Could you check a few things on this model? Use its own coordinates, in mm. Face numbers are marked on the shaded views. A direction names the side the tool comes from. Give positions to 0.01 mm unless a question says otherwise; leave off trailing zeros. Write each loop counter-clockwise with the first axis right and the second up, starting at its lowest first coordinate (ties: lowest second). Pieces come first, ordered by that corner, then holes. Notation, with made-up numbers: M 31.5,70.5 L 40.5,70.5 A19 ccw 40.5,97.5 Z; hole C 69,-26 d9. An arc over 180 degrees is marked long. One line per item, written item: value.
```python
from build123d import *

# Parameters (mm, degrees)
SKETCH2_R          = 3.5
CUT_EXTRUDE1_DEPTH = 10
FILLET1_R          = 2
CUT_EXTRUDE2_START = -10
CUT_EXTRUDE2_DEPTH = 10


with BuildPart() as part:
    # Sketch1 → Revolve1 (revolve)
    with BuildSketch(Plane.XY, mode=Mode.PRIVATE) as revolve1_sk:
        Polygon((-8, 7), (-8, 23), (-4, 23), (-4, 60), (2, 60), (2, 45), (8, 45), (8, 40), (2, 40), (2, 19), (8, 19), (8, 14), (0, 14), (0, 7), align=None)
    revolve(revolve1_sk.sketch.rotate(Axis((0, 0, 0), (1, 0, 0)), 90), axis=Axis((0, 0, 0), (1, 0, 0)))

    # Sketch2 → Cut-Extrude1 (cut)
    with BuildSketch(Plane(origin=(2, 0, 0), x_dir=(0, 0, -1), z_dir=(1, 0, 0))):
        with Locations((0, 51)):
            Circle(SKETCH2_R)
        with Locations((44.167295593, 25.5)):
            Circle(SKETCH2_R)
        with Locations((44.167295593, -25.5)):
            Circle(SKETCH2_R)
        with Locations((0, -51)):
            Circle(SKETCH2_R)
        with Locations((-44.167295593, -25.5)):
            Circle(SKETCH2_R)
        with Locations((-44.167295593, 25.5)):
            Circle(SKETCH2_R)
    extrude(amount=-CUT_EXTRUDE1_DEPTH, mode=Mode.SUBTRACT)

    # Fillet1
    fillet1_edges = [part.edges().sort_by_distance(p)[0] for p in [
        (2, 0, -19),
        (2, 0, -40),
        (-4, 0, -23),
    ]]
    fillet(fillet1_edges, radius=FILLET1_R)

    # Sketch3 → Cut-Extrude2 (cut)
    with BuildSketch(Plane.ZY.offset(4).offset(CUT_EXTRUDE2_START)):
        with BuildLine():
            ThreePointArc((-2.143276082, 59.961707511), (-30, 51.961524227), (-50.856723918, 31.83698529))
            Line((-50.856723918, 31.83698529), (-2.143276082, 59.961707511))
        make_face()
        with BuildLine():
            ThreePointArc((50.856723918, 31.83698529), (30, 51.961524227), (2.143276082, 59.961707511))
            Line((2.143276082, 59.961707511), (50.856723918, 31.83698529))
        make_face()
        with BuildLine():
            ThreePointArc((60, 0), (58.223706512, 14.491376746), (53, 28.124722221))
            Line((53, 28.124722221), (53, -28.124722221))
            ThreePointArc((53, -28.124722221), (58.223706512, -14.491376746), (60, 0))
        make_face()
        with BuildLine():
            Line((50.856723918, -31.83698529), (2.143276082, -59.961707511))
            ThreePointArc((2.143276082, -59.961707511), (30, -51.961524227), (50.856723918, -31.83698529))
        make_face()
        with BuildLine():
            Line((-2.143276082, -59.961707511), (-50.856723918, -31.83698529))
            ThreePointArc((-50.856723918, -31.83698529), (-30, -51.961524227), (-2.143276082, -59.961707511))
        make_face()
        with BuildLine():
            Line((-53, -28.124722221), (-53, 28.124722221))
            ThreePointArc((-53, 28.124722221), (-60, 0), (-53, -28.124722221))
        make_face()
    extrude(amount=CUT_EXTRUDE2_DEPTH, mode=Mode.SUBTRACT)


solid = part.part
```
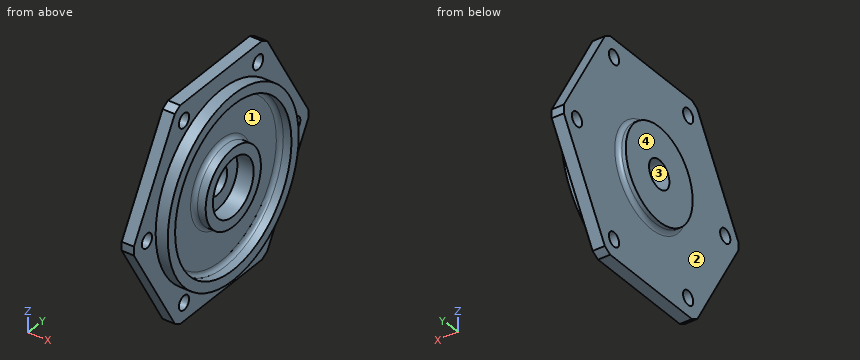
1) We'd pull the mould along Z, two halves only. Please class the marked faces 3 and 4: pulls with the +Z half, pulls with the -Z half, needs draft (parallel to the pull), parting line crosses it, or undercut.
Outcome:
face 3: undercut
face 4: needs draft
2) If we section it at C-C, the plane y = 43.5: Write out the boundary of the cut face in (x, z), then the cut area to 3 significant figures.
Outcome:
outline: M -4,-30.66 L 2,-30.66 L 2,-11.52 L 8,-11.52 L 8,11.52 L 2,11.52 L 2,30.66 L -4,30.66 Z
area: 506 mm^2
3) On a 3-axis mill with a long thin cutter (end or side, diameter ignored), from which of +Z, -Z, +X, -X, +Y, -Y can I reach the whole of each face in a straight line? I mean the marked faces 1 and 2. Say none if no direction works.
Outcome:
face 1: +X
face 2: -X
4) If we section it at D-D, the plane y = -51: Write out the boundary of the cut face in (x, z), then the cut area to 3 significant figures.
Outcome:
outline: M -4,-17.67 L 2,-17.67 L 2,-3.5 L -4,-3.5 Z; M -4,3.5 L 2,3.5 L 2,17.67 L -4,17.67 Z
area: 170 mm^2
5) I'm going to push flat-ended pins straight in: pin 1 (10 mm diameter, centred on y = 26, z = 15.5, fed in from -X); pin 2 (4 mm diameter, centred on y = 32, z = 7.5, fed in from +X); pin 3 (22.5 mm diameter, centred on y = 0, z = 0, fed in from +X). Where does each tip first touch, or does it pass through?
Outcome:
pin 1: stops at x = -4
pin 2: stops at x = 2
pin 3: stops at x = 0
6) Please list where these lines run through material, in increasing order: L1, parallel to Y at x = -2.25, z = 0; L2, parallel to Y at x = 2.25, z = -4; L3, parallel to X at y = -18, z = -29. Write a range as from..to.
Outcome:
L1: y = -60..-54.5, -47.5..-7, 7..47.5, 54.5..60
L2: y = -44.82..-38.76, -19.63..-13.42, 13.42..19.63, 38.76..44.82
L3: x = -4..2
7) If we section it at B-B, the plane z = 0: Give the number of separate pieces and of enclosed holes in the cut face, then the cut area to 3 significant figures.
Outcome:
separate pieces: 4
enclosed holes: 0
area: 777 mm^2
